Check sheet for the modelled part. Datum: model origin and axes. Units: mm. Face numbers are marked on the shaded views. A direction names the side the tool comes from. Round coordinates to 2 decimals unless told otherwise and drop trailing zeros. Write each loop counter-clockwise with the first axis right and the second up, starting at its lowest first coordinate (ties: lowest second). Pieces come first, ordered by that corner, then holes. Notation, with made-up numbers: (-38.5, 16.5) -> (-28.5, 16.5) arc R12 ccw to (-28.5, 33.5) -> close; hole circle Ø2 at (39, -26). An arc over 180 degrees is marked (long way). Write item = value, one per line.
from build123d import *

# Parameters (mm, degrees)
F0_W     = 76.2
F0_H     = 76.2
F1_DEPTH = 25.4
F2_W     = 24.268436
F2_H     = 5.308717
F3_DEPTH = 25.4


with BuildPart() as f1:
    # F0 (on Front) → F1 (new body)
    with BuildSketch(Plane.XZ):
        Rectangle(F0_W, F0_H)
    extrude(amount=F1_DEPTH)

    # F2 (on face) → F3 (join)
    with BuildSketch(Plane(origin=(0, 0, -38.1), x_dir=(1, 0, 0), z_dir=(0, 0, -1))):
        with Locations((-15.167773, 19.149313)):
            Rectangle(F2_W, F2_H)
    extrude(amount=F3_DEPTH)


solid = f1.part
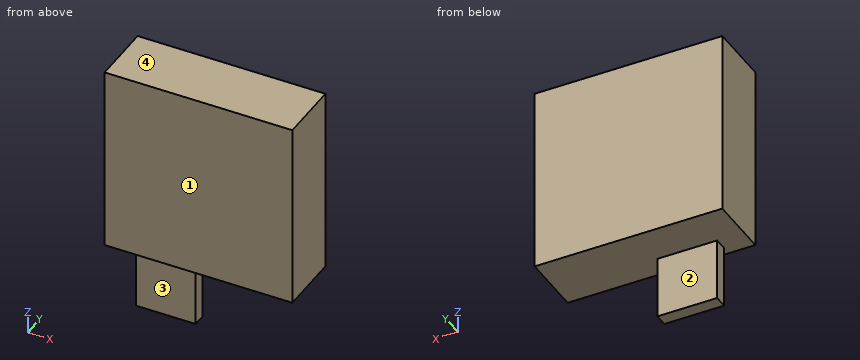
(1) Sectioned sample at A-A on y = -19.75. Enter the section's corners in (x, z), then the cut area to 3 significant figures.
Worked answers:
outline = (-38.1, -38.1) -> (-27.3, -38.1) -> (-27.3, -63.5) -> (-3.03, -63.5) -> (-3.03, -38.1) -> (38.1, -38.1) -> (38.1, 38.1) -> (-38.1, 38.1) -> close
area = 6,420 mm²
(2) Sectioned sample at B-B on x = -20. Enter the section's corners in (y, z).
Worked answers:
outline = (-25.4, -38.1) -> (-21.8, -38.1) -> (-21.8, -63.5) -> (-16.49, -63.5) -> (-16.49, -38.1) -> (0, -38.1) -> (0, 38.1) -> (-25.4, 38.1) -> close
(3) Sectioned sample at D-D on y = -5.25. Enter the section's corners in (x, z), then the cut area to 3 significant figures.
Worked answers:
outline = (-38.1, -38.1) -> (38.1, -38.1) -> (38.1, 38.1) -> (-38.1, 38.1) -> close
area = 5,810 mm²
(4) Go/stop test with flat-tipped pins: P1, Ø7.5, axis at x = -17.5, z = -54.5, coming from the -Y side; P2, Ø5, axis at x = 30.5, y = -16, coming from the -Z side; P3, Ø6, axis at y = -20, z = -57, coming from the -X side. Record where each tip stops, or that it passes through.
Worked answers:
P1 = -21.8
P2 = -38.1
P3 = -27.3
(5) Release check for a two-part mould opening along Z. For the marked faces 3 and 4 record: pulls with the +Z half, pulls with the -Z half, needs draft (parallel to the pull), parting line crosses it, or undercut.
Worked answers:
face_3 = needs draft
face_4 = pulls with the +Z half
(6) Access from +Z, -Z, +X, -X, +Y, -Y to the whole of each face (thin tool, end or side, straight path). Record for the marked faces 1 and 2.
Worked answers:
face_1 = +Z, -Z, +X, -X, -Y
face_2 = -Z, +X, -X, +Y
(7) Material ranges on L1, parallel to Z at x = 2, y = -16.25; L2, parallel to Y at x = -19.5, z = -57.5, recorded low to high. Write a range as [from, to].
Worked answers:
L1 = [-38.1, 38.1]
L2 = [-21.8, -16.49]
(8) Sectioned sample at C-C on z = -52. Enter the section's corners in (x, y).
Worked answers:
outline = (-27.3, -21.8) -> (-3.03, -21.8) -> (-3.03, -16.49) -> (-27.3, -16.49) -> close
